Autodesk Inventor part; units mm, degrees
ref_plane "YZ Plane" through (0, 0, 0) normal (1, 0, 0) x (0, 1, 0)
ref_plane "XZ Plane" through (0, 0, 0) normal (0, 1, 0) x (-1, 0, 0)
ref_plane "XY Plane" through (0, 0, 0) normal (0, 0, 1) x (1, 0, 0)
sketch "Sketch1" plane through (0, 0, 0) normal (0, 0, 1) x (1, 0, 0)
  line L0 (0, 7.5) -> (100, 7.5)
  line L1 (100, 7.5) -> (100, 7.5)
  line L2 (126.4895, 0) -> (0, 0)
  line L3 (0, 0) -> (0, 7.5)
  line L4 (100, 7.5) -> (124.4895, 7.5)
  line L5 (126.4895, 5.5) -> (126.4895, 0)
  arc A0 (126.4895, 5.5) -> (124.4895, 7.5) centre (124.4895, 5.5) ccw
  dimension "d0" = 100
  dimension "d2" = 7.5
  dimension "d8" = 2
revolve "Revolution1" add sketch "Sketch1" angle 360 about axis through (126.4895, 0, 0) along (-1, 0, 0)
sketch "Sketch3" plane through (0, 0, 0) normal (-1, 0, 0) x (0, 0, 1)
  circle A0 centre (0, 0) radius 4.07
  dimension "d9" = 8.14
extrude "Extrusion2" cut sketch "Sketch3" against normal blind 3.2
fillet "Fillet1" radius 1 1 edges at (0, 0, -4.07)
properties part number "axis"
Build history of the part. All positions in model axes, mm. A direction names the side the tool comes from. Give positions to 0.01 mm unless a question says otherwise; leave off trailing zeros. Order: outer loops, then holes, each group sorted by start corner. A loop starts at its lowest first (then second) coordinate and runs counter-clockwise, first axis right, second up. Notation, with made-up numbers: M 71.5,55 L 86.5,55 A9 ccw 86.5,66 Z; hole C 6.5,32 d5. An arc over 180 degrees is marked long. Use one line per item in the form item = value.
1) Two-plate mould, pull along Z, no slides. Class faces 1 (the face through (126.49, 0, 0)), 2 (the face through (3.2, 0, 0)), 3 (the face through (63.116, -7.493, 0.33)): released by +Z, released by -Z, zero draft, split by the parting line, or undercut.
Calculated:
face_1 = zero draft
face_2 = undercut
face_3 = split by the parting line
2) Probe probe 1 along Y at (x, z) = (2.6, 0); probe 2 along X at (y, z) = (-0.75, -2.25); probe 3 along Z at (x, y) = (83.5, 0.5). List the from-to ranges inside material, lowest first.
Calculated:
probe_1 = -7.5 to -4.07, 4.07 to 7.5
probe_2 = 3.2 to 126.49
probe_3 = -7.48 to 7.48
3) Tool access for faces 4 (the face through (0, 2, 5)), 5 (the face through (2.085, 1.223, 3.882)): list every direction of +Z, -Z, +X, -X, +Y, -Y with a clear straight run to the whole face (end or side of a thin tool).
Calculated:
face_4 = +Z, -Z, -X, +Y, -Y
face_5 = -X
4) Drop flat-ended pins along their axis: pin 1 (2 mm diameter, centred on x = 47, z = 4.5, fed in from +Y); pin 2 (1 mm diameter, centred on x = 70, y = 4.5, fed in from -Z). Give the stop position or say it passes through.
Calculated:
pin_1 = 6.63
pin_2 = -6.34
5) Saw through at A-A (x = 72). Give the cut face in (y, z).
Calculated:
outline = C 0,0 d15
